```python
from build123d import *

# Parameters (mm, degrees)
SKETCH2_R           = 2.75
BOSS_EXTRUDE1_DEPTH = 10


# Read off the part's stored shape, not the designer's step: M4 Machine Threads Stud1
with BuildPart() as part:
    # Sketch1 → Revolve1 (revolve)
    with BuildSketch(Plane.XY):
        Polygon((0, 0), (0, 5), (5, 5), (5, 3), (228, 3), (228, 0), align=None)
    revolve(axis=Axis((228, 0, 0), (-1, 0, 0)))

    # Sketch2 → Boss-Extrude1 (add)
    with BuildSketch(Plane(origin=(228, 0, 0), x_dir=(0, 0, -1), z_dir=(1, 0, 0))):
        with Locations(Location((0, 0, 0), (0, 0, 90))):
            Circle(SKETCH2_R)
    extrude(amount=BOSS_EXTRUDE1_DEPTH)

    # M4 Machine Threads Stud1 outline → M4 Machine Threads Stud1 (revolve, cut)
    with BuildSketch(Plane.YX):
        Polygon((2, 237.61), (2, 228), (2.75, 228), (2.75, 238), (1.61, 238), align=None)
    revolve(axis=Axis((0, 0, 0), (1, 0, 0)), mode=Mode.SUBTRACT)


solid = part.part
```
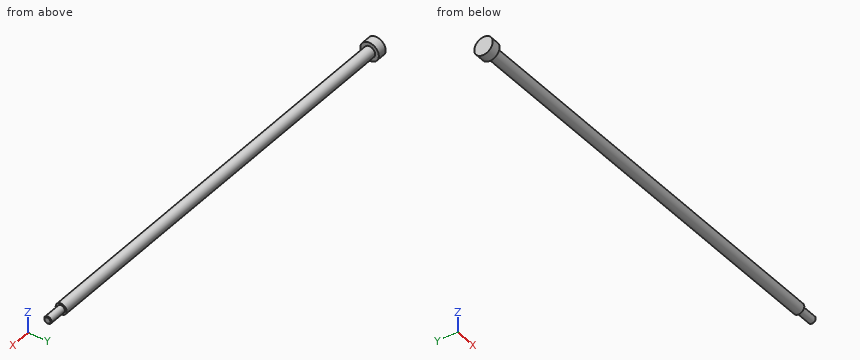
Work out the finished part from the listing and answer in its coordinate system (mm). Round coordinates to 2 decimals unless told otherwise and drop trailing zeros. Write each loop counter-clockwise with the first axis right and the second up, starting at its lowest first coordinate (ties: lowest second). Pieces come first, ordered by that corner, then holes.
1) Consider probe 1 along Y at (x, z) = (190.5, -0.5); probe 2 along X at (y, z) = (0, -3.5). Determine where each line is inside the solid, lowest interval first.
2) A cutting plane is placed at A-A on y = 0. Determine the outline of the cut face in (x, z).
3) A cutting plane is placed at C-C on x = 154. Determine the outline of the cut face in (y, z), and give its area (3 significant figures).
4) Flat-ended cylindrical pins translate along their axes: P1, Ø2, axis at x = 189.5, y = -3, coming from the -Z side; P2, Ø1, axis at x = 212, y = -1.5, coming from the +Z side; P3, Ø5, axis at x = 70.5, z = 3, coming from the -Y side; P4, Ø3, axis at y = 0, z = 3, coming from the +X side. Find the tip coordinate at first contact, or state that the pin passes through.
Entries:
1. probe 1: y = -2.96 to 2.96
1. probe 2: x = 0 to 5
2. outline: (0, -5) - (5, -5) - (5, -3) - (228, -3) - (228, -2) - (237.61, -2) - (238, -1.61) - (238, 1.61) - (237.61, 2) - (228, 2) - (228, 3) - (5, 3) - (5, 5) - (0, 5) - close
3. outline: circle Ø6 at (0, 0)
3. area: 28.3 mm2
4. P1: stops at z = -2.24
4. P2: stops at z = 2.83
4. P3: stops at y = -2.96
4. P4: stops at x = 238
